from build123d import *

# Parameters (mm, degrees)
SKETCH_1_R          = 10.5
EXTRUDE_1_DEPTH     = 2
SKETCH_2_R          = 4
SKETCH_2_R_2        = 3
EXTRUDE_2_DEPTH     = 4
SKETCH_5_R          = 1.5
CUT_EXTRUDE_2_DEPTH = 16.378556499
FILLET_1_R          = 1
SKETCH_6_R          = 3.5
EXTRUDE_3_DEPTH     = 0.5
SKETCH_8_R          = 3
CUT_EXTRUDE_3_DEPTH = 1.5
SKETCH_9_R          = 1
CUT_EXTRUDE_5_DEPTH = 17.015617378


with BuildPart() as part:
    # 草圖1 → 伸長1 (new body)
    with BuildSketch(Plane.XY):
        Circle(SKETCH_1_R)
    extrude(amount=EXTRUDE_1_DEPTH)

    # 草圖2 → 伸長2 (add)
    with BuildSketch(Plane.XY.offset(2)):
        Circle(SKETCH_2_R)
        Circle(SKETCH_2_R_2, mode=Mode.SUBTRACT)
    extrude(amount=EXTRUDE_2_DEPTH)

    # 草圖5 → 除料-伸長2 (cut, through all)
    with BuildSketch(Plane.XY.offset(2)):
        Circle(SKETCH_5_R)
    extrude(amount=-CUT_EXTRUDE_2_DEPTH, mode=Mode.SUBTRACT)

    # 圓角1
    fillet_1_edges = [part.edges().sort_by_distance(p)[0] for p in [
        (-4, 0, 2),
    ]]
    fillet(fillet_1_edges, radius=FILLET_1_R)

    # 草圖6 → 伸長3 (add)
    with BuildSketch(Plane(origin=(0, 0, 0), x_dir=(-1, 0, 0), z_dir=(0, 0, -1))):
        with Locations(Location((0, 0, 0), (0, 0, 180))):
            Circle(SKETCH_6_R)
    extrude(amount=EXTRUDE_3_DEPTH)

    # 草圖8 → 除料-伸長3 (cut)
    with BuildSketch(Plane(origin=(0, 0, -0.5), x_dir=(-1, 0, 0), z_dir=(0, 0, -1))):
        with Locations(Location((0, 0, 0), (0, 0, 180))):
            Circle(SKETCH_8_R)
    extrude(amount=-CUT_EXTRUDE_3_DEPTH, mode=Mode.SUBTRACT)

    # 草圖9 → 除料-伸長5 (cut, through all)
    with BuildSketch(Plane(origin=(0, 0, 0), x_dir=(-1, 0, 0), z_dir=(0, 0, -1))):
        with Locations((8.25, 0)):
            Circle(SKETCH_9_R)
        with Locations((0, -8.25)):
            Circle(SKETCH_9_R)
        with Locations((-8.25, 0)):
            Circle(SKETCH_9_R)
        with Locations((0, 8.25)):
            Circle(SKETCH_9_R)
        with Locations((5.28030303, -6.338840581)):
            Circle(SKETCH_9_R)
        with Locations((-6.338840581, -5.28030303)):
            Circle(SKETCH_9_R)
        with Locations((-5.28030303, 6.338840581)):
            Circle(SKETCH_9_R)
        with Locations((6.338840581, 5.28030303)):
            Circle(SKETCH_9_R)
        with Locations((6.791614908, -3.181818182)):
            Circle(SKETCH_9_R)
        with Locations((-3.181818182, -6.791614908)):
            Circle(SKETCH_9_R)
        with Locations((-6.791614908, 3.181818182)):
            Circle(SKETCH_9_R)
        with Locations((3.181818182, 6.791614908)):
            Circle(SKETCH_9_R)
    extrude(amount=-CUT_EXTRUDE_5_DEPTH, mode=Mode.SUBTRACT)


solid = part.part
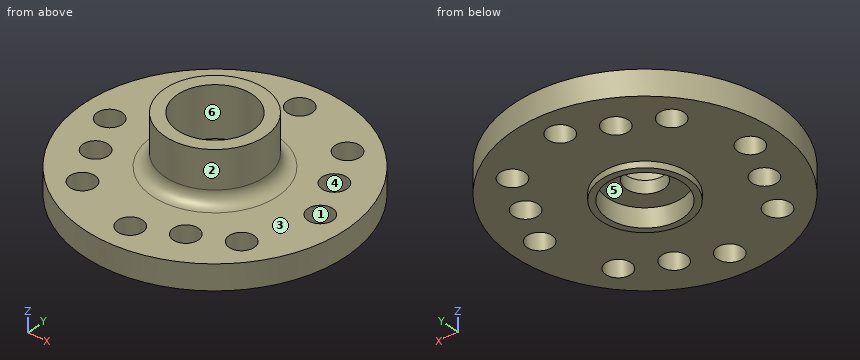
Can you work these out from the model? Positions are in its coordinate system, mm. Face numbers are marked on the shaded views. A direction names the side the tool comes from. Round coordinates to 2 decimals unless told otherwise and drop trailing zeros. Write each loop counter-clockwise with the first axis right and the second up, starting at its lowest first coordinate (ties: lowest second). Pieces come first, ordered by that corner, then holes. Notation, with made-up numbers: (83.25, 76.5) -> (125.25, 76.5) arc R16 ccw to (125.25, 100.5) -> close; hole circle Ø3 at (16.25, -19.5). An arc over 180 degrees is marked (long way). One line per question, with ' | ' between items. Start each with the question number.
1) I need wall thicknesses on line 1 (Y direction, x = 0, z = 0.9); line 2 (Z direction, x = 4.25, y = 4.5); line 3 (Z direction, x = -0.25, y = -3.75). Which ranges of each line are inside material? Lowest first, please. Write a range as [from, to].
2) I'm going to push flat-ended pins straight in: P1, Ø1.2, axis at x = 3.18, y = -6.79, coming from the -Z side; P2, Ø1, axis at x = 2, y = 8.5, coming from the +Z side; P3, Ø2.5, axis at x = 0, y = 8.25, coming from the -Z side; P4, Ø3, axis at x = -0.5, y = 1, coming from the -Z side. Where does each tip first touch, or does it pass through?
3) On a 3-axis mill with a long thin cutter (end or side, diameter ignored), from which of +Z, -Z, +X, -X, +Y, -Y can I reach the whole of each face in a straight line? I mean the marked faces 4, 5 and 6. Say none if no direction works.
4) Suppose I cut it at A-A on x = 0. Count the separate pieces of the cut face and the enclosed holes in it, then the cut area to 3 significant figures.
5) Suppose I cut it at D-D on y = 8.25. Write out the boundary of the cut face in (x, z).
6) Suppose I cut it at B-B on x = 8.5. Write out the boundary of the cut face in (y, z), then the cut area to 3 significant figures.
7) If we mould it in two halves opening along X, with no side actions, what happens to the marked faces 1, 2 and 3? For each: released by +X, released by -X, zero draft, split by the parting line, or undercut.
Return value:
1) line 1: y = [-10.5, -9.25], [-7.25, -3], [3, 7.25], [9.25, 10.5] | line 2: z = [0, 2] | line 3: z = [0, 6]
2) P1: passes through | P2: stops at z = 2 | P3: stops at z = 0 | P4: stops at z = 1
3) face 4: +Z, -Z | face 5: -Z | face 6: +Z
4) separate pieces: 4 | enclosed holes: 0 | area: 33.9 mm2
5) outline: (-6.5, 0) -> (-1, 0) -> (-1, 2) -> (-6.5, 2) -> close; (1, 0) -> (6.5, 0) -> (6.5, 2) -> (1, 2) -> close
6) outline: (-6.16, 0) -> (-0.97, 0) -> (-0.97, 2) -> (-6.16, 2) -> close; (0.97, 0) -> (6.16, 0) -> (6.16, 2) -> (0.97, 2) -> close | area: 20.8 mm2
7) face 1: undercut | face 2: split by the parting line | face 3: zero draft
